Design review of the part built by this model. Coordinates are the model's own, in mm. A direction names the side the tool comes from. Coordinates: 2 decimals unless noted, no trailing zeros. Write each loop counter-clockwise with the first axis right and the second up, starting at its lowest first coordinate (ties: lowest second). Pieces come first, ordered by that corner, then holes.
Q1. Take a section at C-C, the plane x = 10.5. Write out the cut boundary in (y, z), plus the area to 3 significant figures.
Q2. Take a section at B-B, the plane z = 0. Write out the cut boundary in (x, y), plus the area to 3 significant figures.
Q3. For L1, parallel to X at y = 6.5, z = 9; L2, parallel to Y at x = 12, z = 5.5; L3, parallel to Z at x = 16.25, y = 1, list the stretches that pass through material, from the lowest coordinate up.
Q4. Take a section at A-A, the plane x = 2. Write out the cut boundary in (y, z).
Q5. For pin 1 Ø6 at (x, y) = (4.5, 7.5) entering from -Z; pin 2 Ø4 at (x, y) = (6.5, 1) entering from +Z; pin 3 Ø1.5 at (y, z) = (9, 7) entering from +X; pin 4 Ø2 at (y, z) = (-8.5, 8) entering from -X, all flat-tipped, find the tip position at first contact; note any pin that passes through.
Q6. For faces 1 (the flat face through (4.056, -5.012, -7.404)), 2 (the cylindrical face through (17.67, 7.81, -1.73)), 3 (the cylindrical face through (4.056, -7.814, 3.345)), 4 (the flat face through (13.209, 6, 4)), 5 (the flat face through (4.06, 3.91, -8.04)), list the 3-axis set-ups (+Z, -Z, +X, -X, +Y, -Y) from which the entire face can be reached by the end or side of a thin tool; tool diameter is ignored.
Q7. Take a section at D-D, the plane x = 20. Write out the cut boundary in (y, z).
Q8. The part is to be moulded in two halves that separate along X. For faces 6 (the flat face through (8, 8.5, -2.7)), 7 (the cylindrical face through (12.22, 6.64, -1.47)), 8 (the flat face through (4.056, -8.918, 0.639)), say which applies: released by +X, released by -X, zero draft, split by the parting line, or undercut.
from build123d import *

# Parameters (mm, degrees)
EXTRUDE_START   = -8
SKETCH_2_R      = 8.5
EXTRUDE_1_DEPTH = 8
CHAMFER_1_SIZE  = 1


with BuildPart() as part:
    # Sketch 1 → 旋转1 (revolve)
    with BuildSketch(Plane.XY, mode=Mode.PRIVATE) as revolve_1_sk:
        Polygon((0, 0), (0, 8.5), (8, 8.5), (8, 13), (11, 13), (11.209265355, 6.8), (13.209265355, 6.8), (13.209265355, 8), (23, 8), (23, 0), align=None)
    revolve(revolve_1_sk.sketch.rotate(Axis((0, 0, 0), (1, 0, 0)), 90), axis=Axis((0, 0, 0), (1, 0, 0)))

    # 草图2 → 凸台-拉伸1 (add)
    # profile 1 of 7: a face of its own
    with BuildSketch(Plane.ZY.offset(EXTRUDE_START)):
        Polygon((-1.174764966, -9.690972033), (7.805245485, -5.86286232), (8.980010451, 3.828109713), (1.174764966, 9.690972033), (-7.805245485, 5.86286232), (-8.980010451, -3.828109713), align=None)
        Circle(SKETCH_2_R, mode=Mode.SUBTRACT)
    # profile 2 of 7: a face of its own
    with BuildSketch(Plane.ZY.offset(EXTRUDE_START)):
        with BuildLine():
            Line((-7.805245485, 5.86286232), (-8.286430908, 1.893426207))
            ThreePointArc((-8.286430908, 1.893426207), (-6.796266629, 5.104974035), (-4.12702026, 7.430861577))
            Line((-4.12702026, 7.430861577), (-7.805245485, 5.86286232))
        make_face()
    # profile 3 of 7: a face of its own
    with BuildSketch(Plane.ZY.offset(EXTRUDE_START)):
        with BuildLine():
            ThreePointArc((-2.503460259, 8.122972777), (1.022903886, 8.43822657), (4.371804767, 7.289535176))
            Line((4.371804767, 7.289535176), (1.174764966, 9.690972033))
            Line((1.174764966, 9.690972033), (-2.503460259, 8.122972777))
        make_face()
    # profile 4 of 7: a face of its own
    with BuildSketch(Plane.ZY.offset(EXTRUDE_START)):
        with BuildLine():
            ThreePointArc((8.5, 0), (8.499706252, -0.070665642), (8.498825028, -0.141326401))
            Line((8.498825028, -0.141326401), (8.980010451, 3.828109713))
            Line((8.980010451, 3.828109713), (5.78297065, 6.22954657))
            ThreePointArc((5.78297065, 6.22954657), (7.79118895, 3.398142837), (8.5, 0))
        make_face()
    # profile 5 of 7: a face of its own
    with BuildSketch(Plane.ZY.offset(EXTRUDE_START)):
        with BuildLine():
            Line((4.12702026, -7.430861577), (7.805245485, -5.86286232))
            Line((7.805245485, -5.86286232), (8.286430908, -1.893426207))
            ThreePointArc((8.286430908, -1.893426207), (6.796266629, -5.104974035), (4.12702026, -7.430861577))
        make_face()
    # profile 6 of 7: a face of its own
    with BuildSketch(Plane.ZY.offset(EXTRUDE_START)):
        with BuildLine():
            Line((-1.174764966, -9.690972033), (2.503460259, -8.122972777))
            ThreePointArc((2.503460259, -8.122972777), (-1.022903886, -8.43822657), (-4.371804767, -7.289535176))
            Line((-4.371804767, -7.289535176), (-1.174764966, -9.690972033))
        make_face()
    # profile 7 of 7: a face of its own
    with BuildSketch(Plane.ZY.offset(EXTRUDE_START)):
        with BuildLine():
            Line((-8.980010451, -3.828109713), (-5.78297065, -6.22954657))
            ThreePointArc((-5.78297065, -6.22954657), (-7.819170515, -3.333252534), (-8.498825028, 0.141326401))
            Line((-8.498825028, 0.141326401), (-8.980010451, -3.828109713))
        make_face()
    extrude(amount=EXTRUDE_1_DEPTH)

    # 倒角1
    chamfer_1_edges = [part.edges().sort_by_distance(p)[0] for p in [
        (23, 0, -8),
    ]]
    chamfer(chamfer_1_edges, length=CHAMFER_1_SIZE)


solid = part.part
Responses:
1. outline: circle Ø26 at (0, 0)
1. area: 531 mm2
2. outline: (0, -9.19) - (8, -9.19) - (8, -13) - (11, -13) - (11.21, -6.8) - (13.21, -6.8) - (13.21, -8) - (22, -8) - (23, -7) - (23, 7) - (22, 8) - (13.21, 8) - (13.21, 6.8) - (11.21, 6.8) - (11, 13) - (8, 13) - (8, 9.19) - (0, 9.19) - close
2. area: 412 mm2
3. L1: x = 8 to 11.06
3. L2: y = -4 to 4
3. L3: z = -7.94 to 7.94
4. outline: (-9.69, -1.17) - (-7.29, -4.37) arc R8.5 ccw to (-6.23, -5.78) - (-3.83, -8.98) - (0.14, -8.5) arc R8.5 ccw to (1.89, -8.29) - (5.86, -7.81) - (7.43, -4.13) arc R8.5 ccw to (8.12, -2.5) - (9.69, 1.17) - (7.29, 4.37) arc R8.5 ccw to (6.23, 5.78) - (3.83, 8.98) - (-0.14, 8.5) arc R8.5 ccw to (-1.89, 8.29) - (-5.86, 7.81) - (-7.43, 4.13) arc R8.5 ccw to (-8.12, 2.5) - close
5. pin 1: stops at z = -7.97
5. pin 2: stops at z = 13
5. pin 3: stops at x = 11.08
5. pin 4: stops at x = 8
6. face 1: -Z, -X, -Y
6. face 2: +X
6. face 3: +Z, -X, -Y
6. face 4: none
6. face 5: -Z, -X, +Y
7. outline: circle Ø16 at (0, 0)
8. face 6: released by -X
8. face 7: undercut
8. face 8: zero draft
